Can you work these out from the model? Positions are in its coordinate system, mm. A direction names the side the tool comes from. Coordinates: 2 decimals unless noted, no trailing zeros. Order: outer loops, then holes, each group sorted by start corner. A loop starts at its lowest first (then second) coordinate and runs counter-clockwise, first axis right, second up. Notation, with made-up numbers: M 32,84 L 60,84 A20 cw 60,91 Z; hole C 40,50.5 d9. An arc over 180 degrees is marked long. Answer as a JSON object with one key per item and string values.
from build123d import *

# Parameters (mm, degrees)
F0_W     = 1219.2
F0_H     = 152.4
F1_DEPTH = 31.75
F2_W     = 88.9
F2_H     = 152.4
F3_DEPTH = 1.27
F4_DEPTH = 1.27


with BuildPart() as f1:
    # F0 (on Front) → F1 (new body)
    with BuildSketch(Plane.XZ):
        with Locations((-609.6, 76.2)):
            Rectangle(F0_W, F0_H)
    extrude(amount=F1_DEPTH)

    # F2 (on face) → F3 (cut)
    with BuildSketch(Plane.XZ.offset(31.75)):
        with Locations((-996.95, 76.2)):
            Rectangle(F2_W, F2_H)
    extrude(amount=-F3_DEPTH, mode=Mode.SUBTRACT)

    # F2 (on face) → F4 (cut)
    with BuildSketch(Plane.XZ.offset(31.75)):
        with Locations((-222.25, 76.2)):
            Rectangle(F2_W, F2_H)
    extrude(amount=-F4_DEPTH, mode=Mode.SUBTRACT)


solid = f1.part
Item 1: Which directions (+Z, -Z, +X, -X, +Y, -Y) give clear straight access to the entire face, cutting with the end or side of a thin tool? Please do faces 1 (the flat face through (-223, -30.48, 77)), 2 (the flat face through (-614, -31.75, 77)).
Answers follow:
{"face 1": "+Z, -Z, -Y", "face 2": "+Z, -Z, +X, -X, -Y"}
Item 2: If we mould it in two halves opening along X, with no side actions, what happens to faces 3 (the flat face through (-90, -31.75, 77)), 4 (the flat face through (-998, -30.48, 77)), 5 (the flat face through (-1219.2, -16, 75))? For each: pulls with the +X half, pulls with the -X half, needs draft (parallel to the pull), parting line crosses it, or undercut.
Answers follow:
{"face 3": "needs draft", "face 4": "undercut", "face 5": "pulls with the -X half"}
Item 3: I want a section at A-A, the plane x = -241. Write out the boundary of the cut face in (y, z).
Answers follow:
{"outline": "M -30.48,0 L 0,0 L 0,152.4 L -30.48,152.4 Z"}
